Design review of the part built by this model. Coordinates are the model's own, in mm. Face numbers are marked on the shaded views. A direction names the side the tool comes from. Coordinates: 2 decimals unless noted, no trailing zeros. Order: outer loops, then holes, each group sorted by start corner. A loop starts at its lowest first (then second) coordinate and runs counter-clockwise, first axis right, second up. Notation, with made-up numbers: M -22.75,44.5 L -12.75,44.5 A15 ccw -12.75,65.5 Z; hole C 11,-31.75 d5. An arc over 180 degrees is marked long. Use CSV: the item, a comma, the result in double quotes.
Autodesk Inventor part; units mm, degrees
ref_plane "YZ Plane" through (0, 0, 0) normal (1, 0, 0) x (0, 1, 0)
ref_plane "XZ Plane" through (0, 0, 0) normal (0, 1, 0) x (-1, 0, 0)
ref_plane "XY Plane" through (0, 0, 0) normal (0, 0, 1) x (1, 0, 0)
sketch "Skizze1" plane through (0, 0, 0) normal (0, 0, 1) x (1, 0, 0)
  circle A0 centre (0, 0) radius 10 construction
  circle A1 centre (0, 0) radius 11.5 construction
  circle A2 centre (0, 0) radius 8.5 construction
  line L0 (10, 0) -> (8.0902, -5.8779) construction
  line L1 (8.0902, -5.8779) -> (3.0902, -9.5106) construction
  line L2 (3.0902, -9.5106) -> (-3.0902, -9.5106) construction
  line L3 (-3.0902, -9.5106) -> (-8.0902, -5.8779) construction
  line L4 (-8.0902, -5.8779) -> (-10, 0) construction
  line L5 (-10, 0) -> (-8.0902, 5.8779) construction
  line L6 (-8.0902, 5.8779) -> (-3.0902, 9.5106) construction
  line L7 (-3.0902, 9.5106) -> (3.0902, 9.5106) construction
  line L8 (3.0902, 9.5106) -> (8.0902, 5.8779) construction
  line L9 (8.0902, 5.8779) -> (10, 0) construction
  arc A3 (8.0902, 5.8779) -> (10, 0) centre (13.0579, 4.2428) ccw
  arc A4 (8.0902, 5.8779) -> (3.0902, 9.5106) centre (4.7642, 6.5573) ccw
  arc A5 (-3.0902, 9.5106) -> (3.0902, 9.5106) centre (0, 13.7299) ccw
  arc A6 (-3.0902, 9.5106) -> (-8.0902, 5.8779) centre (-4.7642, 6.5573) ccw
  arc A7 (-10, 0) -> (-8.0902, 5.8779) centre (-13.0579, 4.2428) ccw
  arc A8 (-10, 0) -> (-8.0902, -5.8779) centre (-7.7086, -2.5047) ccw
  arc A9 (-3.0902, -9.5106) -> (-8.0902, -5.8779) centre (-8.0703, -11.1078) ccw
  arc A10 (-3.0902, -9.5106) -> (3.0902, -9.5106) centre (0, -8.1053) ccw
  arc A11 (8.0902, -5.8779) -> (3.0902, -9.5106) centre (8.0703, -11.1078) ccw
  arc A12 (8.0902, -5.8779) -> (10, 0) centre (7.7086, -2.5047) ccw
  point P0 (0, -11.5)
  point P1 (10.9371, -3.5537)
  point P2 (6.7595, 9.3037)
  point P3 (-6.7595, 9.3037)
  point P4 (-10.9371, -3.5537)
  dimension "d0" = 20
  dimension "d1" = 23
  dimension "d2" = 17
extrude "Extrusion1" add sketch "Skizze1" along normal blind 10
sketch "Skizze2" plane through (0, 0, 10) normal (0, 0, 1) x (1, 0, 0)
  circle A0 centre (0, 0) radius 5.75 construction
  line L0 (0, 5.75) -> (4.9796, 2.875)
  line L1 (4.9796, 2.875) -> (4.9796, -2.875)
  line L2 (4.9796, -2.875) -> (0, -5.75)
  line L3 (0, -5.75) -> (-4.9796, -2.875)
  line L4 (-4.9796, -2.875) -> (-4.9796, 2.875)
  line L5 (-4.9796, 2.875) -> (0, 5.75)
  dimension "d11" = 11.5
extrude "Extrusion2" cut sketch "Skizze2" against normal blind 4.5
chamfer "Fase1" distance 2.5 angle 45 10 edges at (-8.084, 2.6266, 10) (-10.9371, -3.5537, 10) (-4.9962, -6.8766, 10) (0, -11.5, 10) (4.9962, -6.8766, 10) (10.9371, -3.5537, 10) (8.084, 2.6266, 10) (6.7595, 9.3037, 10) (0, 8.5, 10) (-6.7595, 9.3037, 10)
properties part number "Damper" material "Gummi, Butyl"
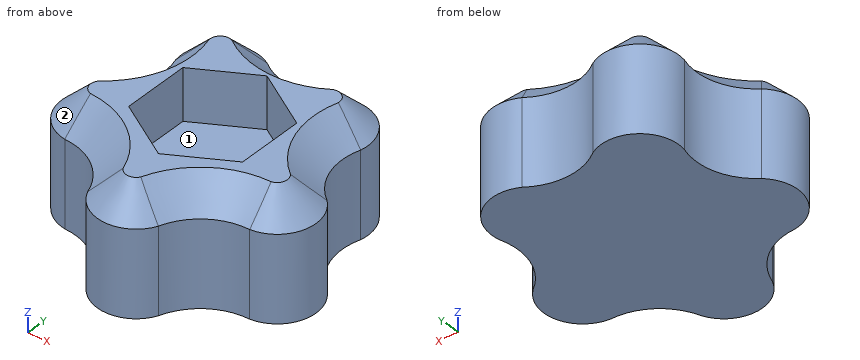
(1) Wall thickness on probe 1 along X at (y, z) = (9.25, 4.5); probe 2 along Z at (x, y) = (3, 3); probe 3 along X at (y, z) = (1.5, 3.5): over which ranges is each line inside the solid? List them lowest first.
The answers:
probe 1,"x = -6.83 to -2.7, 2.7 to 6.83"
probe 2,"z = 0 to 5.5"
probe 3,"x = -8.6 to 8.6"
(2) Add section B-B on z = 2. State the section outline as (x, y) points.
The answers:
outline,"M -10,0 A3.39 ccw -8.09,-5.88 A5.23 cw -3.09,-9.51 A3.39 ccw 3.09,-9.51 A5.23 cw 8.09,-5.88 A3.39 ccw 10,0 A5.23 cw 8.09,5.88 A3.39 ccw 3.09,9.51 A5.23 cw -3.09,9.51 A3.39 ccw -8.09,5.88 A5.23 cw Z"
(3) Add section A-A on z = 8.5. State the section outline as (x, y) points (3 decimals).
The answers:
outline,"M -9.362,-0.772 A2.395 ccw -8.028,-4.878 A6.23 cw -2.158,-9.143 A2.395 ccw 2.158,-9.143 A6.23 cw 8.028,-4.878 A2.395 ccw 9.362,-0.772 A6.23 cw 7.12,6.128 A2.395 ccw 3.628,8.665 A6.23 cw -3.628,8.665 A2.395 ccw -7.12,6.128 A6.23 cw Z; hole M -4.98,-2.875 L 0,-5.75 L 4.98,-2.875 L 4.98,2.875 L 0,5.75 L -4.98,2.875 Z"
(4) Clearance check with flat-ended pins moving along their axes: P1, Ø1.5, axis at y = -4, z = 4.5, coming from the +X side; P2, Ø1.3, axis at y = 0, z = 8.5, coming from the +X side; P3, Ø2, axis at x = 0.5, y = -8, coming from the -Z side; P4, Ø1, axis at y = 3.5, z = 2.5, coming from the -X side. State where each tip first meets the part, or that it passes through.
The answers:
P1,"stops at x = 11.02"
P2,"stops at x = 9.71"
P3,"stops at z = 0"
P4,"stops at x = -7.98"
(5) For the marked faces 1 and 2, list the 3-axis set-ups (+Z, -Z, +X, -X, +Y, -Y) from which the entire face can be reached by the end or side of a thin tool; tool diameter is ignored.
The answers:
face 1,"+Z"
face 2,"+Z, -X"
(6) Add section C-C on z = 6.5. State the section outline as (x, y) points (3 decimals).
The answers:
outline,"M -10,0 A3.395 ccw -8.09,-5.878 A5.23 cw -3.09,-9.511 A3.395 ccw 3.09,-9.511 A5.23 cw 8.09,-5.878 A3.395 ccw 10,0 A5.23 cw 8.09,5.878 A3.395 ccw 3.09,9.511 A5.23 cw -3.09,9.511 A3.395 ccw -8.09,5.878 A5.23 cw Z; hole M -4.98,-2.875 L 0,-5.75 L 4.98,-2.875 L 4.98,2.875 L 0,5.75 L -4.98,2.875 Z"
